```python
from build123d import *

# Parameters (mm, degrees)
BOSS_EXTRUDE1_DEPTH = 1
EXTRUDE_THIN1_DEPTH = 2.5
SKETCH2_R           = 1.5
BOSS_EXTRUDE2_DEPTH = 4


with BuildPart() as part:
    # Sketch1 → Boss-Extrude1 (new body)
    with BuildSketch(Plane.XY):
        with BuildLine():
            Line((-3.9, 0.888819442), (-2.48949833, 16.228906238))
            ThreePointArc((-2.48949833, 16.228906238), (0, 18.5), (2.48949833, 16.228906238))
            Line((2.48949833, 16.228906238), (3.9, 0.888819442))
            ThreePointArc((3.9, 0.888819442), (0, -4), (-3.9, 0.888819442))
        make_face()
    extrude(amount=BOSS_EXTRUDE1_DEPTH)

    # Sketch1_3 → Extrude-Thin1 (add)
    with BuildSketch(Plane.XY):
        with BuildLine():
            Line((-4.394954578, 0.966630363), (-2.987397996, 16.274687485))
            ThreePointArc((-2.987397996, 16.274687485), (0, 19), (2.987397996, 16.274687485))
            Line((2.987397996, 16.274687485), (4.394954578, 0.966630363))
            ThreePointArc((4.394954578, 0.966630363), (0, -4.5), (-4.394954578, 0.966630363))
        make_face()
        with BuildLine():
            Line((-3.9, 0.888819442), (-2.48949833, 16.228906238))
            ThreePointArc((-2.48949833, 16.228906238), (0, 18.5), (2.48949833, 16.228906238))
            Line((2.48949833, 16.228906238), (3.9, 0.888819442))
            ThreePointArc((3.9, 0.888819442), (0, -4), (-3.9, 0.888819442))
        make_face(mode=Mode.SUBTRACT)
    extrude(amount=EXTRUDE_THIN1_DEPTH)

    # Sketch2 → Boss-Extrude2 (add)
    with BuildSketch(Plane(origin=(0, 0, 0), x_dir=(-1, 0, 0), z_dir=(0, 0, -1))):
        with Locations(Location((0, 16, 0), (0, 0, 180))):
            Circle(SKETCH2_R)
    extrude(amount=BOSS_EXTRUDE2_DEPTH)


solid = part.part
```
Part model, mm, in its own coordinate system. A direction names the side the tool comes from. Coordinates: 2 decimals unless noted, no trailing zeros. Order: outer loops, then holes, each group sorted by start corner. A loop starts at its lowest first (then second) coordinate and runs counter-clockwise, first axis right, second up. Notation, with made-up numbers: (86, -17) - (125, -17) arc R16 cw to (125, -9) - close; hole circle Ø9 at (-3.75, 56.25). An arc over 180 degrees is marked (long way). Return JSON: item names as keys, results as strings. Group by question number.
Item 1: Cut at C-C (x = 0). List the corners of the cut face in (y, z).
Item 2: Drill centre lines: probe 1 along X at (y, z) = (0, 1.9); probe 2 along Z at (x, y) = (-0.75, 0); probe 3 along X at (y, z) = (2.25, 1.5). Where is each one in solid material? Low to high. Write a range as from..to.
Item 3: Cut at B-B (y = 0). List the corners of the cut face in (x, z), plus the area to 3 significant figures.
Item 4: Cut at D-D (z = -3). List the corners of the cut face in (x, y), plus the area to 3 significant figures.
Item 5: Pin check, flat tips, straight feed: pin 1 (2 mm diameter, centred on x = 2, z = -0.5, fed in from +Y); pin 2 (2.5 mm diameter, centred on x = -1, y = 1.5, fed in from -Z). Stop position of each tip, or through.
Item 6: Cut at A-A (z = 2). List the corners of the cut face in (x, y), plus the area to 3 significant figures.
Item 7: Pull direction Y, two halves, no side cores. Call faces 1 (the face through (-0.325, 17.464, -1.972)), 2 (the face through (3.7, 6.4, 2.5)), 3 (the face through (3.68, 8.73, 1.23)), 4 (the face through (-3.2, 8.5, 1.7)): pulls with the +Y half, pulls with the -Y half, needs draft (parallel to the pull), parting line crosses it, or undercut.
Item 8: Which spindle directions (+Z, -Z, +X, -X, +Y, -Y) get a long thin tool onto all of the face, cutting with end or side? Do faces 5 (the face through (-0.1, 18.5, 1.7)), 6 (the face through (-3.7, 8.51, 1.23)). Say none if no direction does.
Check values:
{
 "1": {"outline": "(-4.5, 0) - (14.5, 0) - (14.5, -4) - (17.5, -4) - (17.5, 0) - (19, 0) - (19, 2.5) - (18.5, 2.5) - (18.5, 1) - (-4, 1) - (-4, 2.5) - (-4.5, 2.5) - close"},
 "2": {"probe 1": "x = -4.5..-4, 4..4.5", "probe 2": "z = 0..1", "probe 3": "x = -4.28..-3.77, 3.77..4.28"},
 "3": {"outline": "(-4.5, 0) - (4.5, 0) - (4.5, 2.5) - (4, 2.5) - (4, 1) - (-4, 1) - (-4, 2.5) - (-4.5, 2.5) - close", "area": "10.5 mm2"},
 "4": {"outline": "circle Ø3 at (0, 16)", "area": "7.07 mm2"},
 "5": {"pin 1": "stops at y = 18.78", "pin 2": "stops at z = 0"},
 "6": {"outline": "(-4.39, 0.97) arc R4.5 ccw (long way) to (4.39, 0.97) - (2.99, 16.27) arc R3 ccw to (-2.99, 16.27) - close; hole (-3.9, 0.89) arc R4 ccw (long way) to (3.9, 0.89) - (2.49, 16.23) arc R2.5 ccw to (-2.49, 16.23) - close", "area": "27.1 mm2"},
 "7": {"face 1": "parting line crosses it", "face 2": "needs draft", "face 3": "pulls with the +Y half", "face 4": "undercut"},
 "8": {"face 5": "+Z", "face 6": "+Z, -Z, -X, +Y"}
}
